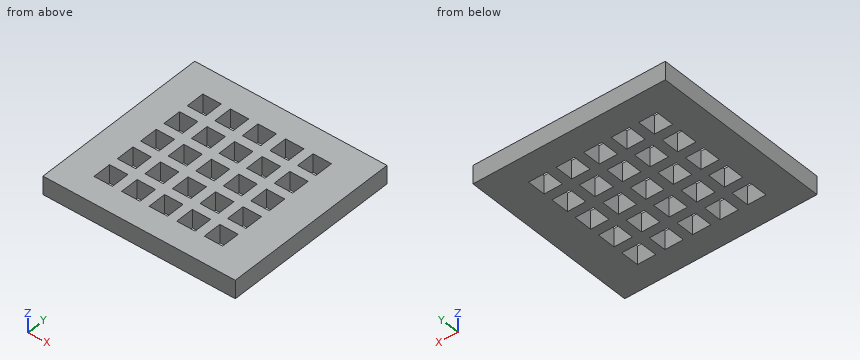
```python
from build123d import *

# Parameters (mm, degrees)
F1_W     = 104.644717
F1_H     = 97.599118
F2_DEPTH = 10
F0_W     = 10
F0_H     = 10
F3_DEPTH = 25


with BuildPart() as f2:
    # F1 (on Top) → F2 (new body)
    with BuildSketch(Plane.XY):
        with Locations((26.015675, 35.25167)):
            Rectangle(F1_W, F1_H)
    extrude(amount=F2_DEPTH)

    # F0 (on Top) → F3 (cut)
    with BuildSketch(Plane.XY):
        with Locations((-5, 5)):
            Rectangle(F0_W, F0_H)
        with Locations((-5, 20)):
            Rectangle(F0_W, F0_H)
        with Locations((-5, 35)):
            Rectangle(F0_W, F0_H)
        with Locations((-5, 50)):
            Rectangle(F0_W, F0_H)
        with Locations((-5, 65)):
            Rectangle(F0_W, F0_H)
        with Locations((10, 5)):
            Rectangle(F0_W, F0_H)
        with Locations((10, 20)):
            Rectangle(F0_W, F0_H)
        with Locations((10, 35)):
            Rectangle(F0_W, F0_H)
        with Locations((10, 50)):
            Rectangle(F0_W, F0_H)
        with Locations((10, 65)):
            Rectangle(F0_W, F0_H)
        with Locations((25, 5)):
            Rectangle(F0_W, F0_H)
        with Locations((25, 20)):
            Rectangle(F0_W, F0_H)
        with Locations((25, 35)):
            Rectangle(F0_W, F0_H)
        with Locations((25, 50)):
            Rectangle(F0_W, F0_H)
        with Locations((25, 65)):
            Rectangle(F0_W, F0_H)
        with Locations((40, 5)):
            Rectangle(F0_W, F0_H)
        with Locations((40, 20)):
            Rectangle(F0_W, F0_H)
        with Locations((40, 35)):
            Rectangle(F0_W, F0_H)
        with Locations((40, 50)):
            Rectangle(F0_W, F0_H)
        with Locations((40, 65)):
            Rectangle(F0_W, F0_H)
        with Locations((55, 5)):
            Rectangle(F0_W, F0_H)
        with Locations((55, 20)):
            Rectangle(F0_W, F0_H)
        with Locations((55, 35)):
            Rectangle(F0_W, F0_H)
        with Locations((55, 50)):
            Rectangle(F0_W, F0_H)
        with Locations((55, 65)):
            Rectangle(F0_W, F0_H)
    extrude(amount=F3_DEPTH, mode=Mode.SUBTRACT)


solid = f2.part
```
Work out the finished part from the listing and answer in its coordinate system (mm). Round coordinates to 2 decimals unless told otherwise and drop trailing zeros. Write each loop counter-clockwise with the first axis right and the second up, starting at its lowest first coordinate (ties: lowest second). Pieces come first, ordered by that corner, then holes. Notation, with made-up numbers: (80, 1) - (139, 1) arc R13 ccw to (139, 13) - close; hole circle Ø5 at (70, 83). An arc over 180 degrees is marked (long way). Return JSON: item names as keys, results as strings. Group by question number.
Q1. This flat-tipped pin is pushed along its axis until it touches: pin 1 Ø10 at (x, y) = (38, 40.5) entering from -Z. Where does it stop, or does it pass through?
Q2. Find the intervals of material crossed by L1, parallel to X at y = 9, z = 9.75; L2, parallel to Y at x = -6, z = 4.25, in increasing order.
Q3. The part is cut by section A-A on y = 7. Write down the section's boundary in (x, z).
Q4. The part is cut by section B-B on x = 56.5. Write down the section's boundary in (y, z).
Q5. The part is cut by section C-C on z = 5.5. Count the separate pieces of the cut face and the enclosed holes in it, then the cut area to 3 significant figures.
Solved:
{
 "1": {"pin 1": "z = 0"},
 "2": {"L1": "-26.31 to -10, 0 to 5, 15 to 20, 30 to 35, 45 to 50, 60 to 78.34", "L2": "-13.55 to 0, 10 to 15, 25 to 30, 40 to 45, 55 to 60, 70 to 84.05"},
 "3": {"outline": "(-26.31, 0) - (-10, 0) - (-10, 10) - (-26.31, 10) - close; (0, 0) - (5, 0) - (5, 10) - (0, 10) - close; (15, 0) - (20, 0) - (20, 10) - (15, 10) - close; (30, 0) - (35, 0) - (35, 10) - (30, 10) - close; (45, 0) - (50, 0) - (50, 10) - (45, 10) - close; (60, 0) - (78.34, 0) - (78.34, 10) - (60, 10) - close"},
 "4": {"outline": "(-13.55, 0) - (0, 0) - (0, 10) - (-13.55, 10) - close; (10, 0) - (15, 0) - (15, 10) - (10, 10) - close; (25, 0) - (30, 0) - (30, 10) - (25, 10) - close; (40, 0) - (45, 0) - (45, 10) - (40, 10) - close; (55, 0) - (60, 0) - (60, 10) - (55, 10) - close; (70, 0) - (84.05, 0) - (84.05, 10) - (70, 10) - close"},
 "5": {"separate pieces": "1", "enclosed holes": "25", "area": "7,710 mm²"}
}
